Autodesk Inventor part; units mm, degrees
ref_plane "YZ Plane" through (0, 0, 0) normal (1, 0, 0) x (0, 1, 0)
ref_plane "XZ Plane" through (0, 0, 0) normal (0, 1, 0) x (-1, 0, 0)
ref_plane "XY Plane" through (0, 0, 0) normal (0, 0, 1) x (1, 0, 0)
sketch "Sketch1" plane through (0, 0, 0) normal (0, 1, 0) x (-1, 0, 0)
  line L0 (0, 0) -> (30, 0)
  line L1 (30, 0) -> (30, -60)
  line L2 (30, -60) -> (0, -60)
  line L3 (0, -60) -> (0, 0)
  dimension "d0" = 30
  dimension "d1" = 60
extrude "Extrusion1" add sketch "Sketch1" along normal blind 14
sketch "Sketch2" plane through (-30, 0, 0) normal (0, 0, 1) x (1, 0, 0)
  line L0 (0, 0) -> (0, 14)
  line L1 (0, 7) -> (10, 7)
  circle A0 centre (10, 7) radius 3
  point P0 (30, 0)
  dimension "d4" = 10
  dimension "d5" = 6
extrude "Extrusion2" add sketch "Sketch2" along normal blind 1
sketch "Sketch3" plane through (-20, 7, 1) normal (0, 0, 1) x (1, 0, 0)
  circle A0 centre (0, 0) radius 4
  point P0 (20, -7)
  dimension "d8" = 8
extrude "Extrusion3" add sketch "Sketch3" along normal blind 1
sketch "Sketch4" plane through (-20, 7, 2) normal (0, 0, 1) x (1, 0, 0)
  circle A0 centre (0, 0) radius 2.5
  point P0 (20, -7)
  dimension "d11" = 5
extrude "Extrusion4" cut sketch "Sketch4" against normal blind 1
sketch "Sketch5" plane through (0, 0, -60) normal (0, 0, -1) x (-1, 0, 0)
  line L0 (30, 0) -> (30, 14)
  line L1 (30, 7) -> (20, 7)
  circle A0 centre (20, 7) radius 3
  point P0 (0, 0)
  dimension "d14" = 10
  dimension "d15" = 6
extrude "Extrusion5" add sketch "Sketch5" along normal blind 1
sketch "Sketch6" plane through (-20, 7, -61) normal (0, 0, -1) x (-1, 0, 0)
  circle A0 centre (0, 0) radius 4.5
  point P0 (-20, -7)
  dimension "d18" = 9
extrude "Extrusion6" add sketch "Sketch6" along normal blind 30
sketch "Sketch7" plane through (-30, 0, -60) normal (-1, 0, 0) x (0, 0, 1)
  line L0 (60, 0) -> (30, 0)
  line L1 (0, 0) -> (60, 0)
  line L2 (30, 0) -> (35, 0)
  line L3 (35, 0) -> (35, 14)
  line L4 (0, 14) -> (60, 14)
  line L5 (35, 14) -> (25, 14)
  line L6 (25, 14) -> (25, 0)
  line L7 (25, 0) -> (30, 0)
  circle A0 centre (30, 7) radius 4.5
  dimension "d21" = 5
  dimension "d22" = 10
  dimension "d23" = 9
extrude "Extrusion7" cut sketch "Sketch7" against normal blind 10
sketch "Sketch8" plane through (-30, 7, -30) normal (-1, 0, 0) x (0, 0, 1)
  circle A0 centre (0, 0) radius 4.5
  point P0 (30, -7)
extrude "Extrusion8" add sketch "Sketch8" along normal blind 10
sketch "Sketch9" plane through (-40, 7, -30) normal (-1, 0, 0) x (0, 0, 1)
  circle A0 centre (0, 0) radius 2
  point P0 (30, -7)
  dimension "d28" = 4
extrude "Extrusion9" add sketch "Sketch9" along normal blind 1
sketch "Sketch10" plane through (-41, 7, -30) normal (-1, 0, 0) x (0, 0, 1)
  circle A0 centre (0, 0) radius 3
  line L0 (0, -3) -> (-2.5981, -1.5)
  line L1 (-2.5981, -1.5) -> (-2.5981, 1.5)
  line L2 (-2.5981, 1.5) -> (0, 3)
  line L3 (0, 3) -> (2.5981, 1.5)
  line L4 (2.5981, 1.5) -> (2.5981, -1.5)
  line L5 (2.5981, -1.5) -> (0, -3)
  point P0 (30, -7)
  dimension "d31" = 6
extrude "Extrusion10" add sketch "Sketch10" along normal blind 1 contours L4 L5 L0 L1 L2 L3
sketch "Sketch11" plane through (-20, 7, -91) normal (0, 0, -1) x (-1, 0, 0)
  line L0 (0, -4.5) -> (0, 4.5)
  circle A0 centre (0, 0) radius 2.5
  point P0 (-20, -7)
  dimension "d34" = 5
extrude "Extrusion11" cut sketch "Sketch11" against normal blind 10
properties part number "vacuumGenerator"
Read the model definition and answer for the solid it produces. Units are mm, in the model's axes. A direction names the side the tool comes from. Coordinates: 2 decimals unless noted, no trailing zeros. Loops run counter-clockwise (first coordinate to the right, second up) from the corner with the lowest first, then second, coordinate; pieces in that order, holes last.
(1) The part is cut by section D-D (z = -77.5). Determine the outline of the cut face in (x, y), and give its area (3 significant figures).
Solution:
outline: circle Ø9 at (-20, 7)
area: 63.6 mm2
(2) Consider line 1 along Z through (x, y) = (-19.5, 9); line 2 along Z through (x, y) = (-9, 4); line 3 along Z through (x, y) = (-29.5, 3). Determine where each line is inside the solid, lowest interval first.
Solution:
line 1: z = -81 to 1
line 2: z = -60 to 0
line 3: z = -60 to -35, -32.06 to -27.94, -25 to 0
(3) Flat-ended cylindrical pins translate along their axes: pin 1 Ø8 at (x, y) = (-19, 6.5) entering from +Z; pin 2 Ø4 at (y, z) = (12, -18) entering from -X; pin 3 Ø4 at (x, y) = (-37.5, 7.5) entering from -Z; pin 4 Ø4.5 at (x, y) = (-20, 7) entering from -Z. Find the tip coordinate at first contact, or state that the pin passes through.
Solution:
pin 1: stops at z = 2
pin 2: stops at x = -30
pin 3: stops at z = -34.5
pin 4: stops at z = -81
(4) A tool of negligible diameter and unlimited length cuts with its end or side. For faces 1 (the face through (-29.86, 8.72, -25.84)), 2 (the face through (-23.2, 9.4, 1.5)), 3 (the face through (-40, 5, -29)), from which of +Z, -Z, +X, -X, +Y, -Y can it reach the whole face along a straight path? Write none if from no direction.
Solution:
face 1: -X
face 2: +Z
face 3: none
(5) The mould has two halves that part along Z. Classify faces 4 (the face through (-15, 0, -30)), 5 (the face through (-20, 10.2, -33.4)), 6 (the face through (-22, 5, -91)): released by +Z, released by -Z, zero draft, split by the parting line, or undercut.
Solution:
face 4: zero draft
face 5: undercut
face 6: released by -Z
(6) The part is cut by section A-A (y = 1). Determine the outline of the cut face in (x, z).
Solution:
outline: (-30, -60) - (0, -60) - (0, 0) - (-30, 0) - (-30, -25) - (-20, -25) - (-20, -35) - (-30, -35) - close
(7) The part is cut by section C-C (x = -35). Determine the outline of the cut face in (y, z).
Solution:
outline: circle Ø9 at (7, -30)
(8) The part is cut by section B-B (z = -31). Determine the outline of the cut face in (x, y), and give its area (3 significant figures).
Solution:
outline: (-42, 4.58) - (-41, 4.58) - (-41, 5.27) - (-40, 5.27) - (-40, 2.61) - (-20, 2.61) - (-20, 0) - (0, 0) - (0, 14) - (-20, 14) - (-20, 11.39) - (-40, 11.39) - (-40, 8.73) - (-41, 8.73) - (-41, 9.42) - (-42, 9.42) - close
area: 464 mm2
